from build123d import *

# Parameters (mm, degrees)
BOSS_EXTRUDE1_DEPTH        = 25.4
SKETCH2_W                  = 38.1
SKETCH2_H                  = 11.1125
BOSS_EXTRUDE2_DEPTH        = 38.1
SKETCH3_W                  = 38.1
SKETCH3_H                  = 11.1125
BOSS_EXTRUDE3_DEPTH        = 38.1
F_0_328IN_DOWEL_HOLE1_D    = 8.3312
F_0_55IN_DOWEL_HOLE2_D     = 13.8938
F_0_55IN_DOWEL_HOLE2_DEPTH = 35.052
F_0_55IN_DOWEL_HOLE2_TIP   = 4.174118634


with BuildPart() as part:
    # Sketch1 → Boss-Extrude1 (new body)
    with BuildSketch(Plane.XY):
        Polygon((0, 0), (0, 22.225), (-62.932032303, 22.225), (6.35, 62.225), (31.75, 62.225), (101.032032303, 22.225), (38.1, 22.225), (38.1, 0), align=None)
    extrude(amount=BOSS_EXTRUDE1_DEPTH)

    # Sketch2 → Boss-Extrude2 (add)
    with BuildSketch(Plane.XY.offset(25.4)):
        with Locations((19.05, 5.55625)):
            Rectangle(SKETCH2_W, SKETCH2_H)
    extrude(amount=BOSS_EXTRUDE2_DEPTH)

    # Sketch3 → Boss-Extrude3 (add)
    with BuildSketch(Plane(origin=(0, 0, 0), x_dir=(-1, 0, 0), z_dir=(0, 0, -1))):
        with Locations((-19.05, 5.55625)):
            Rectangle(SKETCH3_W, SKETCH3_H)
    extrude(amount=BOSS_EXTRUDE3_DEPTH)

    # Ø0.328in Dowel Hole1 (through all)
    with Locations(Plane(origin=(0, 11.1125, 0), x_dir=(1, 0, 0), z_dir=(0, 1, 0))):
        with Locations((19.05, 25.4), (19.05, -50.8)):
            Hole(F_0_328IN_DOWEL_HOLE1_D / 2)

    # Ø0.55in Dowel Hole2
    with Locations(Plane(origin=(0, 62.225, 0), x_dir=(1, 0, 0), z_dir=(0, 1, 0))):
        with Locations((19.05, -12.7)):
            Hole(F_0_55IN_DOWEL_HOLE2_D / 2, depth=F_0_55IN_DOWEL_HOLE2_DEPTH)
            with Locations((0, 0, -(F_0_55IN_DOWEL_HOLE2_DEPTH + F_0_55IN_DOWEL_HOLE2_TIP / 2))):  # 118° drill point
                Cone(0, F_0_55IN_DOWEL_HOLE2_D / 2, F_0_55IN_DOWEL_HOLE2_TIP, mode=Mode.SUBTRACT)


solid = part.part
Read the model definition and answer for the solid it produces. Units are mm, in the model's axes. A direction names the side the tool comes from. Coordinates: 2 decimals unless noted, no trailing zeros. Write each loop counter-clockwise with the first axis right and the second up, starting at its lowest first coordinate (ties: lowest second). Pieces come first, ordered by that corner, then holes. Notation, with made-up numbers: (19, 60) - (25, 60) arc R21 ccw to (25, 89) - close; hole circle Ø5 at (1.5, 1.5). An arc over 180 degrees is marked (long way). One line per question, with ' | ' between items.
Q1. Find section C-C, the plane y = 20.5. Write down the section's boundary in (x, z).
Result set:
outline: (0, 0) - (38.1, 0) - (38.1, 25.4) - (0, 25.4) - close
Q2. Each of these flat-tipped pins is pushed along its axis until it touches: P1, Ø15.5, axis at x = 7.5, y = 47.5, coming from the -Z side; P2, Ø7.5, axis at x = -37.5, z = 15.5, coming from the -Y side (3 decimals); P3, Ø6, axis at y = 13.5, z = -17, coming from the +X side. Where does it stop, or does it pass through?
Result set:
P1: z = 0 | P2: y = 22.225 | P3: x = 38.1
Q3. Consider L1, parallel to Z at x = 19.05, y = 6.5; L2, parallel to Z at x = 19.05, y = 42; L3, parallel to X at y = 8.5, z = -25.4. Determine where each line is inside the solid, lowest interval first. Write a range as [from, to].
Result set:
L1: [-38.1, -29.57], [-21.23, 46.63], [54.97, 63.5] | L2: [0, 5.75], [19.65, 25.4] | L3: [0, 14.88], [23.22, 38.1]
Q4. Find section A-A, the plane z = -25.4. Write down the section's boundary in (x, y), plus the area to 3 significant figures.
Result set:
outline: (0, 0) - (14.88, 0) - (14.88, 11.11) - (0, 11.11) - close; (23.22, 0) - (38.1, 0) - (38.1, 11.11) - (23.22, 11.11) - close | area: 331 mm^2
Q5. For faces 1 (the flat face through (38.1, 8, 13)), 2 (the flat face through (20, 37, 25.4)), 3 (the flat face through (0, 8, 13)), 4 (the flat face through (19, 11.112, -19)), 5 (the flat face through (-28.776, 41.945, 12.522)), determine the directions among +Z, -Z, +X, -X, +Y, -Y from which every point of the face is accessible in a straight line to the end or side of a thin tool.
Result set:
face 1: +Z, -Z, +X, -Y | face 2: +Z, +X, -X, +Y | face 3: +Z, -Z, -X, -Y | face 4: -Z, +X, -X, +Y | face 5: +Z, -Z, -X, +Y
Q6. Find section D-D, the plane y = 44.5. Write down the section's boundary in (x, z).
Result set:
outline: (-24.35, 0) - (62.45, 0) - (62.45, 25.4) - (-24.35, 25.4) - close; hole circle Ø13.89 at (19.05, 12.7)
Q7. Determine the mould class of faces 6 (the flat face through (19, 11.112, 44)), 7 (the cylindrical face through (24.56, 44.45, 16.93)), 8 (the flat face through (65.906, 42.505, 12.522)) for opening direction X: +X half, -X half, draft (parallel to the pull), parting line (faces both ways), or undercut.
Result set:
face 6: draft | face 7: undercut | face 8: +X half
Q8. Find section B-B, the plane x = 10. Write down the section's boundary in (y, z) (1 decimal), plus the area to 3 significant figures.
Result set:
outline: (0, -38.1) - (11.1, -38.1) - (11.1, 0) - (62.2, 0) - (62.2, 25.4) - (11.1, 25.4) - (11.1, 63.5) - (0, 63.5) - close | area: 2,430 mm^2
